Input: part model. Units: mm. Frame: model coordinates. A direction names the side the tool comes from. Give positions to 0.01 mm unless a question says otherwise; leave off trailing zeros. Loops run counter-clockwise (first coordinate to the right, second up) from the corner with the lowest first, then second, coordinate; pieces in that order, holes last. Notation, with made-up numbers: M -17,-18.5 L 26,-18.5 A23 ccw 26,-2.5 Z; hole C 43.25,38.25 d7. An arc over 180 degrees is marked long. Return JSON: item names as keys, results as strings. Group by question number.
```python
from build123d import *

# Parameters (mm, degrees)
BOSS_EXTRUDE1_OUTLINE_W  = 69.85
BOSS_EXTRUDE1_OUTLINE_H  = 10.16
BOSS_EXTRUDE1_DEPTH      = 5.08
SKETCH2_W                = 74.93
SKETCH2_H                = 36.068
BOSS_EXTRUDE2_DEPTH      = 25.4
FILLET1_R                = 15.24
SHELL5_START             = -17.78
SHELL5_DEPTH             = 20.32
SKETCH8_W                = 5.08
SKETCH8_H                = 20.32
CUT_EXTRUDE1_DEPTH       = 39.37
FILLET2_R                = 2.54
FILLET3_R                = 1.27
BOSS_EXTRUDE4_DEPTH      = 0.00254
BOSS_EXTRUDE4_DEPTH_BACK = 26.67
SKETCH4_W                = 20.32
SKETCH4_H                = 13.208
SKETCH9_R                = 3.175
CUT_EXTRUDE2_DEPTH       = 87.597276135
SKETCH10_R               = 5.690074484
CUT_EXTRUDE3_DEPTH       = 6.35
SKETCH11_R               = 1.5875
CUT_EXTRUDE4_DEPTH       = 7.62
SKETCH12_W               = 76.2
SKETCH12_H               = 5.08
CUT_EXTRUDE5_DEPTH       = 2.54
BOSS_EXTRUDE5_DEPTH      = 2.032
SKETCH14_W               = 15.24
SKETCH14_H               = 6.35
CUT_EXTRUDE6_DEPTH       = 2.54
SKETCH16_W               = 15.24
SKETCH16_H               = 8.128
CUT_EXTRUDE8_DEPTH       = 25.4
BOSS_EXTRUDE6_DEPTH      = 2.54


# Read off the part's stored shape, not the designer's step: Boss-Extrude1, Shell5
with BuildPart() as part:
    # Boss-Extrude1 outline → Boss-Extrude1 (new body)
    with BuildSketch(Plane.XY):
        with Locations((34.925, 5.08)):
            Rectangle(BOSS_EXTRUDE1_OUTLINE_W, BOSS_EXTRUDE1_OUTLINE_H)
    extrude(amount=BOSS_EXTRUDE1_DEPTH)

    # Sketch2 → Boss-Extrude2 (add)
    with BuildSketch(Plane.XY.offset(5.08)):
        with Locations((22.225, 25.654)):
            Rectangle(SKETCH2_W, SKETCH2_H)
    extrude(amount=-BOSS_EXTRUDE2_DEPTH)

    # Fillet1
    fillet1_edges = [part.edges().sort_by_distance(p)[0] for p in [
        (59.69, 7.62, -10.16),
        (59.69, 43.688, -7.62),
        (-15.24, 7.62, -7.62),
        (-15.24, 43.688, -7.62),
    ]]
    fillet(fillet1_edges, radius=FILLET1_R)

    # Shell5 outline → Shell5 (cut)
    with BuildSketch(Plane.XY.offset(SHELL5_START)):
        with BuildLine():
            ThreePointArc((-12.7, 22.86), (-8.980256121, 13.879743879), (0, 10.16))
            Line((0, 10.16), (44.45, 10.16))
            Line((44.45, 10.16), (44.45, 7.62))
            ThreePointArc((44.45, 7.62), (48.849409051, 8.268810878), (52.874226968, 10.16))
            ThreePointArc((52.874226968, 10.16), (57.878380747, 15.6533232), (59.69, 22.86))
            Line((59.69, 22.86), (59.69, 28.448))
            ThreePointArc((59.69, 28.448), (55.226307345, 39.224307345), (44.45, 43.688))
            Line((44.45, 43.688), (44.45, 41.148))
            Line((44.45, 41.148), (0, 41.148))
            ThreePointArc((0, 41.148), (-8.980256121, 37.428256121), (-12.7, 28.448))
            Line((-12.7, 28.448), (-12.7, 22.86))
        make_face()
    extrude(amount=SHELL5_DEPTH, mode=Mode.SUBTRACT)

    # Sketch8 → Cut-Extrude1 (cut)
    with BuildSketch(Plane(origin=(59.69, 0, 0), x_dir=(0, 0, -1), z_dir=(1, 0, 0))):
        with Locations((20.32, 25.654)):
            Rectangle(SKETCH8_W, SKETCH8_H)
    extrude(amount=-CUT_EXTRUDE1_DEPTH, mode=Mode.SUBTRACT)

    # Fillet2
    fillet2_edges = [part.edges().sort_by_distance(p)[0] for p in [
        (20.32, 15.494, -19.05),
        (20.32, 35.814, -19.05),
    ]]
    fillet(fillet2_edges, radius=FILLET2_R)

    # Fillet3
    fillet3_edges = [part.edges().sort_by_distance(p)[0] for p in [
        (57.791650722, 35.814, -19.05),
        (57.791650722, 15.494, -19.05),
    ]]
    fillet(fillet3_edges, radius=FILLET3_R)

    # Sketch4 → Boss-Extrude4 (add, two sides: drawn at the far end of the back side and taken through both)
    with BuildSketch(Plane.XY.offset(5.08).offset(-BOSS_EXTRUDE4_DEPTH_BACK)):
        with Locations((34.925, 1.016)):
            Rectangle(SKETCH4_W, SKETCH4_H)
    extrude(amount=BOSS_EXTRUDE4_DEPTH + BOSS_EXTRUDE4_DEPTH_BACK)

    # Sketch9 → Cut-Extrude2 (cut, through all)
    with BuildSketch(Plane.XY.offset(5.08254)):
        with Locations((34.925, 0.254)):
            Circle(SKETCH9_R)
    extrude(amount=-CUT_EXTRUDE2_DEPTH, mode=Mode.SUBTRACT)

    # Sketch10 → Cut-Extrude3 (cut)
    with BuildSketch(Plane.XY.offset(5.08)):
        with Locations((5.133620521, 35.306)):
            Circle(SKETCH10_R)
    extrude(amount=-CUT_EXTRUDE3_DEPTH, mode=Mode.SUBTRACT)

    # Sketch11 → Cut-Extrude4 (cut)
    with BuildSketch(Plane.XY.offset(5.08)):
        with Locations((6.35, 5.08)):
            Circle(SKETCH11_R)
        with Locations((63.5, 5.08)):
            Circle(SKETCH11_R)
    extrude(amount=-CUT_EXTRUDE4_DEPTH, mode=Mode.SUBTRACT)

    # Sketch12 → Cut-Extrude5 (cut)
    with BuildSketch(Plane.XY.offset(5.08)):
        with Locations((30.48, 33.782)):
            Rectangle(SKETCH12_W, SKETCH12_H)
    extrude(amount=-CUT_EXTRUDE5_DEPTH, mode=Mode.SUBTRACT)

    # Sketch13 → Boss-Extrude5 (add)
    with BuildSketch(Plane.XY.offset(-17.78)):
        with BuildLine():
            Line((44.45, 41.148), (44.45, 43.688))
            ThreePointArc((44.45, 43.688), (51.108835279, 42.156300869), (56.429175518, 37.869090909))
            ThreePointArc((56.429175518, 37.869090909), (56.573269297, 36.52909706), (55.430910891, 35.814))
            Line((55.430910891, 35.814), (44.45, 35.814))
            Line((44.45, 35.814), (44.45, 41.148))
        make_face()
        with BuildLine():
            Line((44.45, 7.62), (44.45, 15.494))
            Line((44.45, 15.494), (55.430910891, 15.494))
            ThreePointArc((55.430910891, 15.494), (56.573269297, 14.77890294), (56.429175518, 13.438909091))
            ThreePointArc((56.429175518, 13.438909091), (51.108835279, 9.151699131), (44.45, 7.62))
        make_face()
    extrude(amount=BOSS_EXTRUDE5_DEPTH)

    # Sketch14 → Cut-Extrude6 (cut)
    with BuildSketch(Plane.XZ.offset(5.588)):
        with Locations((34.925, 1.90754)):
            Rectangle(SKETCH14_W, SKETCH14_H)
    extrude(amount=-CUT_EXTRUDE6_DEPTH, mode=Mode.SUBTRACT)

    # Sketch16 → Cut-Extrude8 (cut)
    with BuildSketch(Plane.XY.offset(5.08254)):
        with Locations((34.925, 1.016)):
            Rectangle(SKETCH16_W, SKETCH16_H)
    extrude(amount=-CUT_EXTRUDE8_DEPTH, mode=Mode.SUBTRACT)

    # Sketch17 → Boss-Extrude6 (add)
    with BuildSketch(Plane.XY.offset(5.08)):
        with BuildLine():
            Line((44.45, 43.688), (0, 43.688))
            ThreePointArc((0, 43.688), (-7.491923652, 41.719348085), (-13.048284332, 36.322))
            Line((-13.048284332, 36.322), (-7.62, 36.322))
            Line((-7.62, 36.322), (-0.465012494, 36.322))
            ThreePointArc((-0.465012494, 36.322), (5.133620521, 40.996074484), (10.732253536, 36.322))
            Line((10.732253536, 36.322), (57.498284332, 36.322))
            ThreePointArc((57.498284332, 36.322), (51.941923652, 41.719348085), (44.45, 43.688))
        make_face()
    extrude(amount=BOSS_EXTRUDE6_DEPTH)


solid = part.part
```
Item 1: Pull-direction query (X, two-part tool) for faces 5 (the face through (27, 18, 5.08)), 6 (the face through (37.86, -0.96, -20.94)), 7 (the face through (-12.7, 26, -8)), 8 (the face through (33, 3, -20.317)); classes: pulls with the +X half, pulls with the -X half, needs draft (parallel to the pull), parting line crosses it, or undercut.
Item 2: Reachability of faces 1 (the face through (42.545, 1, -8)), 2 (the face through (43, 15.494, -19)), 3 (the face through (44.45, 13, -17)), 4 (the face through (-3, 31.242, 4)) from +Z, -Z, +X, -X, +Y, -Y: full face, straight path, thin tool, end or side. Return the list, or none.
Item 3: Section A-A, the plane x = 63.5. Return loops of the section in (y, z).
Item 4: First-contact query: pin 1 Ø1.3 at (y, z) = (9, -2.5) entering from +X; pin 2 Ø3 at (y, z) = (26.5, -10.5) entering from +X; pin 3 Ø1.6 at (y, z) = (13, -17) entering from -X. Flat tips, straight axial feed; report the tip coordinate or a pass-through.
Item 5: Section C-C, the plane y = 16.5. Return loops of the section in (x, z).
Item 6: Material intervals for line 1 (X direction, y = 5, z = -16.75) (3 decimals); line 2 (Y direction, x = 27, z = -0.5); line 3 (Z direction, x = -8, y = 18), sorted ascending. Write a range as from..to.
Item 7: Section B-B, the plane z = -9.25. Return loops of the section in (x, y) (3 decimals), then the cut area to 3 significant figures.
Item 8: Section D-D, the plane y = -1. Return loops of the section in (x, z) (3 decimals).
Answer below:
{
 "1": {"face 5": "needs draft", "face 6": "undercut", "face 7": "pulls with the +X half", "face 8": "undercut"},
 "2": {"face 1": "+Z", "face 2": "-Z, +X", "face 3": "none", "face 4": "+Z, +X"},
 "3": {"outline": "M 0,0 L 3.49,0 L 3.49,5.08 L 0,5.08 Z; M 6.67,0 L 10.16,0 L 10.16,5.08 L 6.67,5.08 Z"},
 "4": {"pin 1": "x = 44.45", "pin 2": "x = -12.7", "pin 3": "x = -12.25"},
 "5": {"outline": "M -13.85,-20.32 L 20.84,-20.32 L 20.84,-17.78 L -10.99,-17.78 L -10.99,2.54 L 58.3,2.54 L 58.3,5.08 L -13.85,5.08 Z"},
 "6": {"line 1": "24.765..27.305, 42.545..45.085", "line 2": "-5.59..10.16, 41.15..43.69", "line 3": "-20.32..-17.78, 2.54..5.08"},
 "7": {"outline": "M -15.24,22.86 A15.24 ccw 0,7.62 L 24.765,7.62 L 24.765,-5.588 L 45.085,-5.588 L 45.085,7.62 L 44.45,7.62 L 44.45,10.16 L 0,10.16 A12.7 cw -12.7,22.86 L -12.7,28.448 A12.7 cw 0,41.148 L 44.45,41.148 L 44.45,43.688 L 0,43.688 A15.24 ccw -15.24,28.448 Z; hole M 27.305,-3.048 L 42.545,-3.048 L 42.545,5.08 L 27.305,5.08 Z", "area": "496 mm^2"},
 "8": {"outline": "M 24.765,-21.59 L 32.008,-21.59 L 32.008,-20.317 L 27.305,-20.317 L 27.305,5.083 L 24.765,5.083 Z; M 37.842,-21.59 L 45.085,-21.59 L 45.085,5.083 L 42.545,5.083 L 42.545,-20.317 L 37.842,-20.317 Z"}
}
